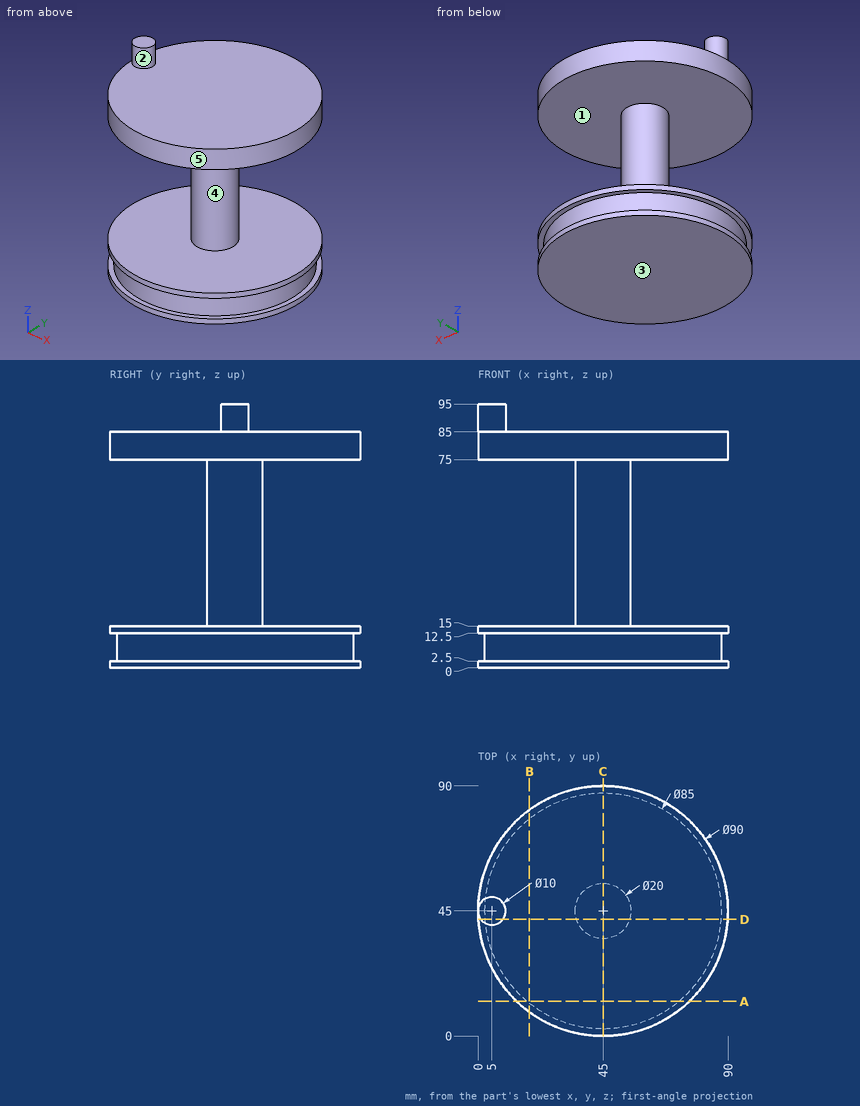
Geometry check sheet. Reference: drawing and pictorial views, mm from the part's lowest x, y, z. A direction names the side the tool comes from. Give positions to 0.01 mm unless a question says otherwise; leave off trailing zeros. Loops run counter-clockwise (first coordinate to the right, second up) from the corner with the lowest first, then second, coordinate; pieces in that order, holes last.
1. Mould release check, pull along Z, two halves, no side actions. Record for the marked faces 1, 2 and 3: released by +Z, released by -Z, zero draft, split by the parting line, or undercut.
2. Section check A-A, the plane y = 12.5. Enter the section's corners in (x, z).
3. Thickness scan on line 1 (Z direction, x = 57, y = 77.5); line 2 (Z direction, x = 51, y = 51); line 3 (Y direction, x = 61, z = 8). Record the ranges inside material, lowest first.
4. Go/stop test with flat-tipped pins: pin 1 Ø8 at (x, z) = (49.5, 41.5) entering from -Y; pin 2 Ø2 at (y, z) = (39, 10.5) entering from +X; pin 3 Ø6 at (y, z) = (36.5, 23) entering from +X. Record where each tip stops, or that it passes through.
5. Section check C-C, the plane x = 45. Enter the section's corners in (y, z).
6. Section check D-D, the plane y = 42. Enter the section's corners in (x, z), then the cut area to 3 significant figures.
7. Set-up check for the marked faces 4 and 5: record each of +Z, -Z, +X, -X, +Y, -Y from which the full face is reachable in a straight line by a thin tool's end or side.
8. Section check B-B, the plane x = 18.5. Enter the section's corners in (y, z), then the cut area to 3 significant figures.
Geometry says:
1. face 1: undercut
1. face 2: zero draft
1. face 3: released by -Z
2. outline: (13.88, 0) - (76.12, 0) - (76.12, 2.5) - (72.39, 2.5) - (72.39, 12.5) - (76.12, 12.5) - (76.12, 15) - (13.88, 15) - (13.88, 12.5) - (17.61, 12.5) - (17.61, 2.5) - (13.88, 2.5) - close; (13.88, 75) - (76.12, 75) - (76.12, 85) - (13.88, 85) - close
3. line 1: z = 0 to 15, 75 to 85
3. line 2: z = 0 to 85
3. line 3: y = 5.63 to 84.37
4. pin 1: stops at y = 35.01
4. pin 2: stops at x = 87.2
4. pin 3: stops at x = 53.35
5. outline: (0, 0) - (90, 0) - (90, 2.5) - (87.5, 2.5) - (87.5, 12.5) - (90, 12.5) - (90, 15) - (55, 15) - (55, 75) - (90, 75) - (90, 85) - (0, 85) - (0, 75) - (35, 75) - (35, 15) - (0, 15) - (0, 12.5) - (2.5, 12.5) - (2.5, 2.5) - (0, 2.5) - close
6. outline: (0.1, 0) - (89.9, 0) - (89.9, 2.5) - (87.39, 2.5) - (87.39, 12.5) - (89.9, 12.5) - (89.9, 15) - (54.54, 15) - (54.54, 75) - (89.9, 75) - (89.9, 85) - (9, 85) - (9, 95) - (1, 95) - (1, 85) - (0.1, 85) - (0.1, 75) - (35.46, 75) - (35.46, 15) - (0.1, 15) - (0.1, 12.5) - (2.61, 12.5) - (2.61, 2.5) - (0.1, 2.5) - close
6. area: 3,420 mm2
7. face 4: none
7. face 5: +Z, -Z
8. outline: (8.63, 0) - (81.37, 0) - (81.37, 2.5) - (78.23, 2.5) - (78.23, 12.5) - (81.37, 12.5) - (81.37, 15) - (8.63, 15) - (8.63, 12.5) - (11.77, 12.5) - (11.77, 2.5) - (8.63, 2.5) - close; (8.63, 75) - (81.37, 75) - (81.37, 85) - (8.63, 85) - close
8. area: 1,760 mm2
